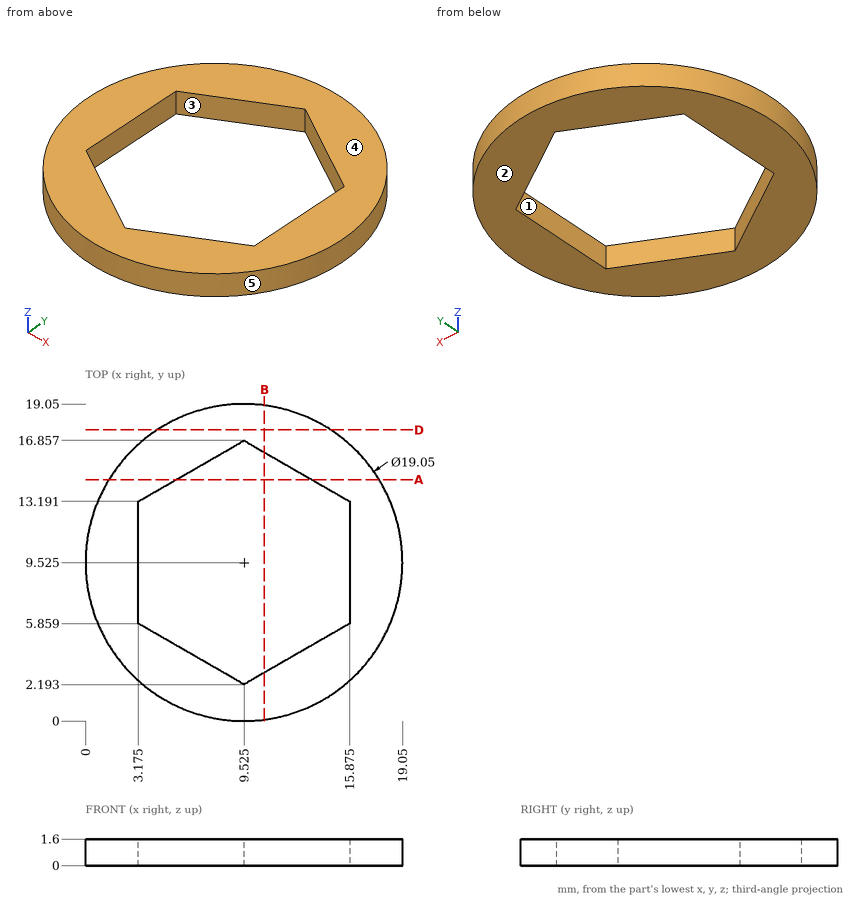
Drawing for the job (mm, zero at the part's lowest x, y, z). A direction names the side the tool comes from. Round coordinates to 2 decimals unless told otherwise and drop trailing zeros. Write each loop counter-clockwise with the first axis right and the second up, starting at its lowest first coordinate (ties: lowest second). Pieces come first, ordered by that corner, then holes. Notation, with made-up numbers: M 46,69 L 100,69 A22 ccw 100,79 Z; hole C -19,-8.75 d5. An arc over 180 degrees is marked long. Answer as a JSON object with one key per item and string values. Group by question number.
(1) Cut at D-D (y = 17.5). Give the cut face in (x, z), and give its area (3 significant figures).
(2) Drill centre lines: L1, parallel to Y at x = 13.5, z = 1.2; L2, parallel to X at y = 13.5, z = 1; L3, parallel to X at y = 6.25, z = 1.3 (1 decimal). Where is each one in solid material? Low to high.
(3) Cut at B-B (x = 10.75). Give the cut face in (y, z).
(4) Flat gauge pin, fed straight in: pin 1 (0.8 mm diameter, centred on y = 11, z = 1, fed in from +X). Where does the tip first touch, or does it go through?
(5) Which spindle directions (+Z, -Z, +X, -X, +Y, -Y) get a long thin tool onto all of the face, cutting with end or side? Do the marked faces 1 and 2. Say none if no direction does.
(6) Cut at A-A (y = 14.5). Give the cut face in (x, z), and give its area (3 significant figures).
(7) Mould opens along X. For the marked faces 3, 4 and 5 say: pulls with the +X half, pulls with the -X half, needs draft (parallel to the pull), parting line crosses it, or undercut.
Responses:
{
 "1": {"outline": "M 4.32,0 L 14.73,0 L 14.73,1.6 L 4.32,1.6 Z", "area": "16.7 mm2"},
 "2": {"L1": "y = 0.87 to 4.49, 14.56 to 18.18", "L2": "x = 0.87 to 3.71, 15.34 to 18.18", "L3": "x = 0.6 to 3.2, 15.9 to 18.5"},
 "3": {"outline": "M 0.08,0 L 2.9,0 L 2.9,1.6 L 0.08,1.6 Z; M 16.15,0 L 18.97,0 L 18.97,1.6 L 16.15,1.6 Z"},
 "4": {"pin 1": "stops at x = 18.99"},
 "5": {"face 1": "+Z, -Z", "face 2": "-Z, +X, -X, +Y, -Y"},
 "6": {"outline": "M 1.4,0 L 5.44,0 L 5.44,1.6 L 1.4,1.6 Z; M 13.61,0 L 17.65,0 L 17.65,1.6 L 13.61,1.6 Z", "area": "12.9 mm2"},
 "7": {"face 3": "undercut", "face 4": "needs draft", "face 5": "parting line crosses it"}
}
